Check sheet for the modelled part. Datum: model origin and axes. Units: mm. A direction names the side the tool comes from. Coordinates: 2 decimals unless noted, no trailing zeros. Loops run counter-clockwise (first coordinate to the right, second up) from the corner with the lowest first, then second, coordinate; pieces in that order, holes last. Notation, with made-up numbers: M 55,63 L 79,63 A19 cw 79,73 Z; hole C 18.5,39 d10. An arc over 180 degrees is marked long. Answer in a Markdown table with one row per item. Add a question column.
```python
from build123d import *

# Parameters (mm, degrees)
F0_W     = 67.8
F0_H     = 4
F1_DEPTH = 4
F0_W_2   = 23.9
F0_H_2   = 80
F2_DEPTH = 4
F0_R     = 2
F0_R_2   = 25.25
F3_DEPTH = 2


with BuildPart() as f1:
    # F0 (on Front) → F1 (new body)
    with BuildSketch(Plane.XZ):
        Polygon((-32.1510285139, 39.2757860942), (-32.1510285139, -24.6242139058), (-32.1510285139, -28.6242139058), (35.6489714861, -28.6242139058), (35.6489714861, 39.2757860942), align=None)
        Polygon((31.6489714861, 35.2757860942), (31.6489714861, -24.6242139058), (-23.1510285139, -24.6242139058), (-28.1510285139, -24.6242139058), (-28.1510285139, 35.2757860942), align=None, mode=Mode.SUBTRACT)
        with Locations((1.7489714861, -30.6242139058)):
            Rectangle(F0_W, F0_H)
    extrude(amount=F1_DEPTH)

    # F0 (on Front) → F2 (join)
    with BuildSketch(Plane.XZ):
        Polygon((-32.1510285139, 39.2757860942), (-32.1510285139, -24.6242139058), (-32.1510285139, -28.6242139058), (35.6489714861, -28.6242139058), (35.6489714861, 39.2757860942), align=None)
        Polygon((31.6489714861, 35.2757860942), (31.6489714861, -24.6242139058), (-23.1510285139, -24.6242139058), (-28.1510285139, -24.6242139058), (-28.1510285139, 35.2757860942), align=None, mode=Mode.SUBTRACT)
        with Locations((1.7489714861, -30.6242139058)):
            Rectangle(F0_W, F0_H)
        with BuildLine():
            Line((35.6489714861, -32.6242139058), (-32.1510285139, -32.6242139058))
            Line((-32.1510285139, -32.6242139058), (-32.1510285139, -142.6242139058))
            Line((-32.1510285139, -142.6242139058), (-15.2010285139, -142.6242139058))
            Line((-15.2010285139, -142.6242139058), (-15.2010285139, -132.6242139058))
            ThreePointArc((-15.2010285139, -132.6242139058), (-18.7365624198, -131.1597478117), (-20.2010285139, -127.6242139058))
            Line((-20.2010285139, -127.6242139058), (-20.2010285139, -47.6242139058))
            ThreePointArc((-20.2010285139, -47.6242139058), (-18.7365624198, -44.0886799999), (-15.2010285139, -42.6242139058))
            Line((-15.2010285139, -42.6242139058), (18.6989714861, -42.6242139058))
            ThreePointArc((18.6989714861, -42.6242139058), (22.234505392, -44.0886799999), (23.6989714861, -47.6242139058))
            Line((23.6989714861, -47.6242139058), (23.6989714861, -127.6242139058))
            ThreePointArc((23.6989714861, -127.6242139058), (22.234505392, -131.1597478117), (18.6989714861, -132.6242139058))
            Line((18.6989714861, -132.6242139058), (18.6989714861, -142.6242139058))
            Line((18.6989714861, -142.6242139058), (35.6489714861, -142.6242139058))
            Line((35.6489714861, -142.6242139058), (35.6489714861, -32.6242139058))
        make_face()
        with BuildLine():
            Line((-15.2010285139, -132.6242139058), (-15.2010285139, -142.6242139058))
            Line((-15.2010285139, -142.6242139058), (1.7489714861, -142.6242139058))
            Line((1.7489714861, -142.6242139058), (18.6989714861, -142.6242139058))
            Line((18.6989714861, -142.6242139058), (18.6989714861, -132.6242139058))
            ThreePointArc((18.6989714861, -132.6242139058), (15.1634375802, -131.1597478117), (13.6989714861, -127.6242139058))
            Line((13.6989714861, -127.6242139058), (-10.2010285139, -127.6242139058))
            ThreePointArc((-10.2010285139, -127.6242139058), (-11.665494608, -131.1597478117), (-15.2010285139, -132.6242139058))
        make_face()
        with Locations((1.7489714861, -87.6242139058)):
            Rectangle(F0_W_2, F0_H_2)
        with BuildLine():
            ThreePointArc((-15.2010285139, -42.6242139058), (-11.665494608, -44.0886799999), (-10.2010285139, -47.6242139058))
            Line((-10.2010285139, -47.6242139058), (13.6989714861, -47.6242139058))
            ThreePointArc((13.6989714861, -47.6242139058), (15.1634375802, -44.0886799999), (18.6989714861, -42.6242139058))
            Line((18.6989714861, -42.6242139058), (-15.2010285139, -42.6242139058))
        make_face()
    extrude(amount=F2_DEPTH)

    # F0 (on Front) → F3 (join)
    with BuildSketch(Plane.XZ):
        Polygon((-23.1510285139, -24.6242139058), (31.6489714861, -24.6242139058), (31.6489714861, 35.2757860942), (-28.1510285139, 35.2757860942), (-28.1510285139, -24.6242139058), align=None)
        with BuildLine():
            ThreePointArc((-21.1510285139, -19.6242139058), (-21.7368149515, -21.0384274682), (-23.1510285139, -21.6242139058))
            ThreePointArc((-23.1510285139, -21.6242139058), (-24.5652420763, -18.2100003434), (-21.1510285139, -19.6242139058))
        make_face(mode=Mode.SUBTRACT)
        with Locations((-23.1510285139, 30.1757860942)):
            Circle(F0_R, mode=Mode.SUBTRACT)
        with Locations((26.6489714861, -19.6242139058)):
            Circle(F0_R, mode=Mode.SUBTRACT)
        with Locations((1.7489714861, 5.3257860942)):
            Circle(F0_R_2, mode=Mode.SUBTRACT)
        with Locations((26.6489714861, 30.1757860942)):
            Circle(F0_R, mode=Mode.SUBTRACT)
    extrude(amount=F3_DEPTH)


solid = f1.part
```
Q1. Cross-section at D-D (x = 7.5). Record the cut outline in (y, z), plus the area to 3 significant figures.
Q2. Cross-section at B-B (y = -2.7). Record the cut outline in (x, z).
Q3. Cross-section at C-C (z = -7.5). Record the cut outline in (x, y), plus the area to 3 significant figures.
Q4. Cross-section at A-A (z = -86). Record the cut outline in (x, y).
Q5. Go/stop test with a flat-tipped pin: pin 1 (18 mm diameter, centred on x = -12.5, z = 18, fed in from -Y). Record where the tip stops, or that it passes through.
Q6. Thickness scan on L1, parallel to X at y = -3.3, z = -56; L2, parallel to Z at x = 13, y = -3.3; L3, parallel to X at y = -3.7, z = 17.5. Record the ranges inside material, lowest first.
Q7. Mould release check, pull along Z, two halves, no side actions. Record for faces 4 (the face through (2, -2, 39.276)), 5 (the face through (-21.304, -0.986, 29.41)), 6 (the face through (1, -2, -142.624)), 7 (the face through (1, -4, -71)): released by +Z, released by -Z, zero draft, split by the parting line, or undercut.
Q8. Access from +Z, -Z, +X, -X, +Y, -Y to the whole of each face (thin tool, end or side, straight path). Record for faces 1 (the face through (-25, -2, 6)), 2 (the face through (23.699, -2, -87)), 3 (the face through (1, 0, -50)).
Answer key:
| question | item | result |
|---|---|---|
| 1 | outline | M -4,-142.62 L 0,-142.62 L 0,-19.26 L -2,-19.26 L -2,-24.62 L -4,-24.62 Z; M -4,35.28 L -2,35.28 L -2,29.91 L 0,29.91 L 0,39.28 L -4,39.28 Z |
| 1 | area | 509 mm^2 |
| 2 | outline | M -32.15,-142.62 L 35.65,-142.62 L 35.65,39.28 L -32.15,39.28 Z; hole M -28.15,-24.62 L 31.65,-24.62 L 31.65,35.28 L -28.15,35.28 Z; hole M -20.2,-127.62 A5 ccw -10.2,-127.62 L -10.2,-47.62 A5 ccw -20.2,-47.62 Z; hole M 13.7,-127.62 A5 ccw 23.7,-127.62 L 23.7,-47.62 A5 ccw 13.7,-47.62 Z |
| 3 | outline | M -32.15,-4 L -28.15,-4 L -28.15,-2 L -20,-2 L -20,0 L -32.15,0 Z; M 23.5,-2 L 31.65,-2 L 31.65,-4 L 35.65,-4 L 35.65,0 L 23.5,0 Z |
| 3 | area | 64.6 mm^2 |
| 4 | outline | M -32.15,-4 L -20.2,-4 L -20.2,0 L -32.15,0 Z; M -10.2,-4 L 13.7,-4 L 13.7,0 L -10.2,0 Z; M 23.7,-4 L 35.65,-4 L 35.65,0 L 23.7,0 Z |
| 5 | pin 1 | y = -2 |
| 6 | L1 | -32.15 to -20.2, -10.2 to 13.7, 23.7 to 35.65 |
| 6 | L2 | -142.62 to -24.62, 35.28 to 39.28 |
| 6 | L3 | -32.15 to -28.15, 31.65 to 35.65 |
| 7 | face 4 | released by +Z |
| 7 | face 5 | undercut |
| 7 | face 6 | released by -Z |
| 7 | face 7 | zero draft |
| 8 | face 1 | -Y |
| 8 | face 2 | +Y, -Y |
| 8 | face 3 | +Z, -Z, +X, -X, +Y |
